from build123d import *

# Parameters (mm, degrees)
SKETCH011_W     = 39.1
SKETCH011_H     = 44.6
SKETCH011_R     = 1.6
PAD007_DEPTH    = 1.6
SKETCH012_R     = 16
PAD008_DEPTH    = 16.5
SKETCH013_R     = 3
SKETCH013_R_2   = 1.6
PAD009_DEPTH    = 4
CHAMFER001_SIZE = 1


with BuildPart() as part:
    # Sketch011 → Pad007 (new body)
    with BuildSketch(Plane.XZ):
        Rectangle(SKETCH011_W, SKETCH011_H)
        with Locations((-15.95, 13.3)):
            Circle(SKETCH011_R, mode=Mode.SUBTRACT)
        with Locations((16.05, 13.3)):
            Circle(SKETCH011_R, mode=Mode.SUBTRACT)
        with Locations((16.05, -18.7)):
            Circle(SKETCH011_R, mode=Mode.SUBTRACT)
        with Locations((-15.95, -18.7)):
            Circle(SKETCH011_R, mode=Mode.SUBTRACT)
    extrude(amount=PAD007_DEPTH)

    # Sketch012 (on Face10 of Pad007) → Pad008 (join)
    with BuildSketch(Plane.XZ.offset(1.6)):
        with Locations((0, -2.7)):
            Circle(SKETCH012_R)
    extrude(amount=PAD008_DEPTH)

    # Sketch013 (on Face4 of Pad008) → Pad009 (join)
    with BuildSketch(Plane(origin=(0, 0, 0), x_dir=(1, 0, 0), z_dir=(0, 1, 0))):
        with Locations((-15.95, 18.7)):
            Circle(SKETCH013_R)
        with Locations((-15.95, 18.7)):
            Circle(SKETCH013_R_2, mode=Mode.SUBTRACT)
        with Locations((16.05, 18.7)):
            Circle(SKETCH013_R)
        with Locations((16.05, 18.7)):
            Circle(SKETCH013_R_2, mode=Mode.SUBTRACT)
        with Locations((16.05, -13.3)):
            Circle(SKETCH013_R)
        with Locations((16.05, -13.3)):
            Circle(SKETCH013_R_2, mode=Mode.SUBTRACT)
        with Locations((-15.95, -13.3)):
            Circle(SKETCH013_R)
        with Locations((-15.95, -13.3)):
            Circle(SKETCH013_R_2, mode=Mode.SUBTRACT)
    extrude(amount=PAD009_DEPTH)

    # Chamfer001
    chamfer001_edges = [part.edges().sort_by_distance(p)[0] for p in [
        (-16, -18.1, -2.7),
    ]]
    chamfer(chamfer001_edges, length=CHAMFER001_SIZE)


with BuildPart() as part_1:
    # Body008 placement: moved
    add(part.part.moved(Location((-20, -18.1, -102.9))))


with BuildPart() as part_2:
    # Clone placement: moved
    add(part_1.part.moved(Location((40, 0, 0))))


solid = part_2.part
Geometry check sheet. Reference: the model listing, model coordinates, mm. A direction names the side the tool comes from. Give positions to 0.01 mm unless a question says otherwise; leave off trailing zeros. Write each loop counter-clockwise with the first axis right and the second up, starting at its lowest first coordinate (ties: lowest second). Pieces come first, ordered by that corner, then holes.
1) Go/stop test with flat-tipped pins: pin 1 Ø3 at (y, z) = (-28, -99) entering from +X; pin 2 Ø10 at (y, z) = (-30, -111) entering from -X (3 decimals); pin 3 Ø1 at (x, z) = (29.5, -108) entering from +Y. Record where each tip stops, or that it passes through.
Values follow:
pin 1: stops at x = 35.17
pin 2: stops at x = 4.005
pin 3: stops at y = -18.1
2) Cross-section at C-C (y = -27). Record the boundary of the cut face in (x, z), plus the area to 3 significant figures.
Values follow:
outline: circle Ø32 at (20, -105.6)
area: 804 mm2
3) Cross-section at A-A (z = -105.6). Record the boundary of the cut face in (x, y), plus the area to 3 significant figures.
Values follow:
outline: (0.45, -19.7) - (4, -19.7) - (4, -35.2) - (5, -36.2) - (35, -36.2) - (36, -35.2) - (36, -19.7) - (39.55, -19.7) - (39.55, -18.1) - (0.45, -18.1) - close
area: 590 mm2
4) Thickness scan on line 1 (X direction, y = -17.3, z = -121.6); line 2 (Z direction, x = 36.05, y = -16.65); line 3 (Y direction, x = 19, z = -110.5). Record the ranges inside material, lowest first.
Values follow:
line 1: x = 1.05 to 2.45, 5.65 to 7.05, 33.05 to 34.45, 37.65 to 39.05
line 2: z = -124.6 to -123.2, -120 to -118.6, -92.6 to -91.2, -88 to -86.6
line 3: y = -36.2 to -18.1
5) Cross-section at B-B (x = 20). Record the boundary of the cut face in (y, z), plus the area to 3 significant figures.
Values follow:
outline: (-36.2, -120.6) - (-35.2, -121.6) - (-19.7, -121.6) - (-19.7, -125.2) - (-18.1, -125.2) - (-18.1, -80.6) - (-19.7, -80.6) - (-19.7, -89.6) - (-35.2, -89.6) - (-36.2, -90.6) - close
area: 598 mm2
6) Release check for a two-part mould opening along X. For faces 4 (the face through (20, -36.2, -105)), 5 (the face through (0.45, -19, -103)), 6 (the face through (36.79, -16.86, -91.02)) record: released by +X, released by -X, zero draft, split by the parting line, or undercut.
Values follow:
face 4: zero draft
face 5: released by -X
face 6: undercut
7) Set-up check for faces 1 (the face through (38.91, -16.13, -90.5)), 2 (the face through (36.79, -16.86, -123.02)), 3 (the face through (16.53, -27.34, -121.22)): record each of +Z, -Z, +X, -X, +Y, -Y from which the full face is reachable in a straight line by a thin tool's end or side.
Values follow:
face 1: +Y
face 2: +Y, -Y
face 3: -Y
